The listing builds one solid part. Answer for the finished solid, in the listing's coordinates (mm). A direction names the side the tool comes from. Coordinates: 2 decimals unless noted, no trailing zeros. Loops run counter-clockwise (first coordinate to the right, second up) from the corner with the lowest first, then second, coordinate; pieces in that order, holes last. Notation, with made-up numbers: (-34, 3.5) - (19, 3.5) arc R21 cw to (19, 24.5) - close; hole circle Ø6 at (-25, 30). An arc over 180 degrees is marked (long way). Put each result on its own line as item: value.
```python
from build123d import *

# Parameters (mm, degrees)
BOSS_EXTRUDE1_DEPTH = 3.175


with BuildPart() as part:
    # Sketch2 → Boss-Extrude1 (new body)
    with BuildSketch(Plane.XY):
        with BuildLine():
            Line((19.538461538, 19.538461538), (31.75, 19.538461538))
            ThreePointArc((31.75, 19.538461538), (51.288461538, 0), (31.75, -19.538461538))
            Line((31.75, -19.538461538), (19.538461538, -19.538461538))
            Line((19.538461538, -19.538461538), (19.538461538, -31.75))
            ThreePointArc((19.538461538, -31.75), (0, -51.288461538), (-19.538461538, -31.75))
            Line((-19.538461538, -31.75), (-19.538461538, -19.538461538))
            Line((-19.538461538, -19.538461538), (-31.75, -19.538461538))
            ThreePointArc((-31.75, -19.538461538), (-51.288461538, 0), (-31.75, 19.538461538))
            Line((-31.75, 19.538461538), (-19.538461538, 19.538461538))
            Line((-19.538461538, 19.538461538), (-19.538461538, 31.75))
            ThreePointArc((-19.538461538, 31.75), (0, 51.288461538), (19.538461538, 31.75))
            Line((19.538461538, 31.75), (19.538461538, 19.538461538))
        make_face()
        with BuildLine():
            Line((-31.75, 12.211538462), (-19.538461538, 12.211538462))
            Line((-19.538461538, 12.211538462), (-19.538461538, 6.35))
            Line((-19.538461538, 6.35), (-31.75, 6.35))
            ThreePointArc((-31.75, 6.35), (-38.1, 0), (-31.75, -6.35))
            Line((-31.75, -6.35), (-15.755245836, -6.35))
            ThreePointArc((-15.755245836, -6.35), (-10.895166245, -5.383270063), (-6.774989715, -2.630256121))
            Line((-6.774989715, -2.630256121), (2.630256121, 6.774989715))
            ThreePointArc((2.630256121, 6.774989715), (8.652052588, 10.798625477), (15.755245836, 12.211538462))
            Line((15.755245836, 12.211538462), (31.75, 12.211538462))
            ThreePointArc((31.75, 12.211538462), (43.961538462, 0), (31.75, -12.211538462))
            Line((31.75, -12.211538462), (19.538461538, -12.211538462))
            Line((19.538461538, -12.211538462), (19.538461538, -6.35))
            Line((19.538461538, -6.35), (31.75, -6.35))
            ThreePointArc((31.75, -6.35), (38.1, 0), (31.75, 6.35))
            Line((31.75, 6.35), (15.755245836, 6.35))
            ThreePointArc((15.755245836, 6.35), (10.895166245, 5.383270063), (6.774989715, 2.630256121))
            Line((6.774989715, 2.630256121), (-2.630256121, -6.774989715))
            ThreePointArc((-2.630256121, -6.774989715), (-8.652052588, -10.798625477), (-15.755245836, -12.211538462))
            Line((-15.755245836, -12.211538462), (-31.75, -12.211538462))
            ThreePointArc((-31.75, -12.211538462), (-43.961538462, 0), (-31.75, 12.211538462))
        make_face(mode=Mode.SUBTRACT)
        with BuildLine():
            Line((-6.35, -31.75), (-6.35, -19.538461538))
            Line((-6.35, -19.538461538), (-12.211538462, -19.538461538))
            Line((-12.211538462, -19.538461538), (-12.211538462, -31.75))
            ThreePointArc((-12.211538462, -31.75), (0, -43.961538462), (12.211538462, -31.75))
            Line((12.211538462, -31.75), (12.211538462, -0.488461538))
            Line((12.211538462, -0.488461538), (6.35, -6.35))
            Line((6.35, -6.35), (6.35, -31.75))
            ThreePointArc((6.35, -31.75), (0, -38.1), (-6.35, -31.75))
        make_face(mode=Mode.SUBTRACT)
        with BuildLine():
            Line((0, 25.4), (0, 19.538461538))
            ThreePointArc((0, 19.538461538), (8.634861655, 40.384861655), (-12.211538462, 31.75))
            Line((-12.211538462, 31.75), (-12.211538462, 0.488461538))
            Line((-12.211538462, 0.488461538), (-6.35, 6.35))
            Line((-6.35, 6.35), (-6.35, 31.75))
            ThreePointArc((-6.35, 31.75), (4.490128061, 36.240128061), (0, 25.4))
        make_face(mode=Mode.SUBTRACT)
    extrude(amount=BOSS_EXTRUDE1_DEPTH)


solid = part.part
```
1) Each of these flat-tipped pins is pushed along its axis until it touches: pin 1 (1 mm diameter, centred on x = -34, z = 2.5, fed in from -Y); pin 2 (1.6 mm diameter, centred on y = -16.5, z = 2, fed in from -X); pin 3 (1 mm diameter, centred on x = -27, z = 1.5, fed in from +Y). Where does it stop, or does it pass through?
Found:
pin 1: stops at y = -19.46
pin 2: stops at x = -43.38
pin 3: stops at y = 19.54
2) For a pull along Y with two mould halves and no side action, classify faces 5 (the face through (38.1, -0.1, 1.6)), 6 (the face through (-51.284, -0.43, 1.565)), 7 (the face through (19.538, 26, 2)) as pulls with the +Y half, pulls with the -Y half, needs draft (parallel to the pull), parting line crosses it, or undercut.
Found:
face 5: undercut
face 6: parting line crosses it
face 7: needs draft
3) Straight lines are drawn through the part: L1, parallel to X at y = 31.75, z = 1.2; L2, parallel to X at y = -35, z = 2.1; L3, parallel to Y at x = 9.5, z = 1.35. For each, find the intervals that lie inside material, in ascending order. Write a range as [from, to].
Found:
L1: x = [-19.54, -12.21], [-6.35, 6.35], [12.21, 19.54]
L2: x = [-19.27, -11.77], [-5.46, 5.46], [11.77, 19.27]
L3: y = [-48.82, -39.42], [-3.2, 4.7], [11.13, 24.08], [39.42, 48.82]
4) The part is cut by section C-C (y = -8). Give the vertices of the cut face in (x, z) (3 decimals).
Found:
outline: (-49.576, 0) - (-40.976, 0) - (-40.976, 3.175) - (-49.576, 3.175) - close; (-3.982, 0) - (6.35, 0) - (6.35, 3.175) - (-3.982, 3.175) - close; (12.212, 0) - (19.538, 0) - (19.538, 3.175) - (12.212, 3.175) - close; (40.976, 0) - (49.576, 0) - (49.576, 3.175) - (40.976, 3.175) - close
5) The part is cut by section B-B (y = 36). Give the vertices of the cut face in (x, z) (3 decimals).
Found:
outline: (-19.071, 0) - (-11.448, 0) - (-11.448, 3.175) - (-19.071, 3.175) - close; (-4.718, 0) - (4.718, 0) - (4.718, 3.175) - (-4.718, 3.175) - close; (11.448, 0) - (19.071, 0) - (19.071, 3.175) - (11.448, 3.175) - close
6) The part is cut by section D-D (z = 2.6). State how many separate pieces and enclosed holes the cut face has, and give its area (3 significant figures).
Found:
separate pieces: 1
enclosed holes: 3
area: 4,110 mm^2
7) For faces 1 (the face through (0.43, -51.284, 1.565)), 2 (the face through (-26, 12.212, 2)), 3 (the face through (19.538, -26, 2)), 4 (the face through (-19.538, 26, 2)), determine the directions among +Z, -Z, +X, -X, +Y, -Y from which every point of the face is accessible in a straight line to the end or side of a thin tool.
Found:
face 1: +Z, -Z, -Y
face 2: +Z, -Z
face 3: +Z, -Z, +X, -Y
face 4: +Z, -Z, -X, +Y
8) The part is cut by section A-A (x = -23). Give the vertices of the cut face in (y, z) (3 decimals).
Found:
outline: (-19.538, 0) - (-12.212, 0) - (-12.212, 3.175) - (-19.538, 3.175) - close; (-6.35, 0) - (6.35, 0) - (6.35, 3.175) - (-6.35, 3.175) - close; (12.212, 0) - (19.538, 0) - (19.538, 3.175) - (12.212, 3.175) - close
